Source: CAD feature listing. Evaluate the final solid. Frame: model axes, mm. Give positions to 0.01 mm unless a question says otherwise; leave off trailing zeros. Order: outer loops, then holes, each group sorted by start corner. A loop starts at its lowest first (then second) coordinate and runs counter-clockwise, first axis right, second up.
```python
from build123d import *

# Parameters (mm, degrees)
SKETCH1_R           = 51.029755332
SKETCH1_R_2         = 50.895830663
BOSS_EXTRUDE1_DEPTH = 20
CUT_EXTRUDE1_DEPTH  = 50
CUT_EXTRUDE3_DEPTH  = 50
CUT_EXTRUDE4_DEPTH  = 50


with BuildPart() as part:
    # Sketch1 → Boss-Extrude1 (new body)
    with BuildSketch(Plane(origin=(0, 0, 0), x_dir=(1, 0, 0), z_dir=(0, 1, 0))):
        with Locations(Location((0, 0, 0), (0, 0, 270))):
            Circle(SKETCH1_R)
        with Locations(Location((0, 0, 0), (0, 0, 270))):
            Circle(SKETCH1_R_2, mode=Mode.SUBTRACT)
    extrude(amount=BOSS_EXTRUDE1_DEPTH)

    # Sketch2 → Cut-Extrude1 (cut)
    with BuildSketch(Plane(origin=(0, 0, 0), x_dir=(1, 0, 0), z_dir=(0, 1, 0))):
        with BuildLine():
            add(Edge.make_bspline(
                [(-34.904731033, -39.559214609), (-30.458455569, -39.265509231), (-8.75106143, -27.58858136), (20.545320777, -14.807136755), (86.675168203, -3.797801784), (38.172145901, 77.469799439), (-39.909980954, 55.809798543), (-65.468102513, 4.660444989), (-50.700851491, -40.602650978), (-34.904731033, -39.559214609)],
                knots=[0, 0, 0, 0, 0.04430768, 0.194241153, 0.328566983, 0.483905616, 0.753189396, 0.842589722, 1, 1, 1, 1], degree=3))
        make_face()
    extrude(amount=CUT_EXTRUDE1_DEPTH, mode=Mode.SUBTRACT)

    # Sketch3 → Cut-Extrude3 (cut)
    with BuildSketch(Plane(origin=(0, 0, 0), x_dir=(1, 0, 0), z_dir=(0, 1, 0))):
        with BuildLine():
            add(Edge.make_bspline(
                [(15.246268895, -30.627230393), (8.812696929, -41.78541341), (-4.179204183, -74.113546423), (71.751860115, -51.38349092), (57.353322601, 23.43159241), (26.480816992, -11.142386759), (15.246268895, -30.627230393)],
                knots=[0, 0, 0, 0, 0.165808592, 0.474148196, 0.71045873, 1, 1, 1, 1], degree=3))
        make_face()
    extrude(amount=CUT_EXTRUDE3_DEPTH, mode=Mode.SUBTRACT)

    # Sketch4 → Cut-Extrude4 (cut)
    with BuildSketch(Plane(origin=(0, 0, 0), x_dir=(1, 0, 0), z_dir=(0, 1, 0))):
        with BuildLine():
            add(Edge.make_bspline(
                [(-9.67297834, -44.564169781), (-11.510509193, -47.228479243), (-7.545033393, -65.726006155), (26.778755679, -53.527914946), (4.528101436, -45.351564648), (-7.606259285, -41.56755118), (-9.67297834, -44.564169781)],
                knots=[0, 0, 0, 0, 0.198613527, 0.560569713, 0.776614167, 1, 1, 1, 1], degree=3))
        make_face()
    extrude(amount=CUT_EXTRUDE4_DEPTH, mode=Mode.SUBTRACT)


solid = part.part
```
1) Material intervals for L1, parallel to Z at x = -28.5, y = 6; L2, parallel to X at y = 19.25, z = 40.5; L3, parallel to Z at x = -28.75, y = 1.25, sorted ascending.
Report:
L1: z = 42.17 to 42.33
L2: x = -31.04 to -30.82
L3: z = 42 to 42.16
2) Section query B-B, the plane z = 47. Return the cut outline in (x, y).
Report:
outline: (-19.88, 0) - (-19.53, 0) - (-19.53, 20) - (-19.88, 20) - close
3) Pin query (flat end, axial travel): pin 1 (2 mm diameter, centred on x = -16, y = 13, fed in from +Z); pin 2 (4 mm diameter, centred on x = -26, z = 40.5, fed in from -Y); pin 3 (12 mm diameter, centred on x = -22, y = 9.5, fed in from -Z); pin 4 (1.5 mm diameter, centred on x = -22, y = 11, fed in from -Z). Return the tip coordinate at first contact, or that it passes through.
Report:
pin 1: stops at z = 48.78
pin 2: passes through
pin 3: stops at z = 42.5
pin 4: stops at z = 45.53
4) Section query A-A, the plane x = -24.25. Return the cut outline in (y, z).
Report:
outline: (0, 44.75) - (20, 44.75) - (20, 44.9) - (0, 44.9) - close
